The listing builds one solid part. Answer for the finished solid, in the listing's coordinates (mm). Round coordinates to 2 decimals unless told otherwise and drop trailing zeros. Write each loop counter-clockwise with the first axis right and the second up, starting at its lowest first coordinate (ties: lowest second). Pieces come first, ordered by that corner, then holes. Notation, with made-up numbers: M 10,89 L 21,89 A20 cw 21,126 Z; hole C 89,31 d5. An arc over 180 degrees is marked long. Write each question's results on one line, items separated by ' | '.
from build123d import *

# Parameters (mm, degrees)
F0_W     = 152.4
F0_H     = 152.4
F0_R     = 12.7
F1_DEPTH = 152.4
F2_R     = 15.0984188398
F2_R_2   = 23.2988824092
F2_R_3   = 22.4609439984
F2_R_4   = 13.2743249865
F3_DEPTH = 152.401


# Not quite as in the source:
# - the program builds the solid bodies; features that only make, move or delete a surface that nothing else refers to are left out


with BuildPart() as f1:
    # F0 (on Top) → F1 (new body)
    with BuildSketch(Plane.XY):
        Rectangle(F0_W, F0_H)
        Circle(F0_R, mode=Mode.SUBTRACT)
    extrude(amount=F1_DEPTH)

    # F2 (on face) → F3 (cut, through all)
    with BuildSketch(Plane.XZ.offset(76.2)):
        with Locations((-40.0141887367, 122.3329827189)):
            Circle(F2_R)
        with Locations((36.8730016053, 114.2153069377)):
            Circle(F2_R_2)
        with Locations((50.8471243083, 33.929079771)):
            Circle(F2_R_3)
        with Locations((-34.4802364707, 44.915728271)):
            Circle(F2_R_4)
    extrude(amount=-F3_DEPTH, mode=Mode.SUBTRACT)


solid = f1.part
1) Section D-D (x = 53.5) is taken. Determine the outline of the cut face in (y, z).
Return value:
outline: M -76.2,0 L 76.2,0 L 76.2,11.63 L -76.2,11.63 Z; M -76.2,56.23 L 76.2,56.23 L 76.2,97.89 L -76.2,97.89 Z; M -76.2,130.54 L 76.2,130.54 L 76.2,152.4 L -76.2,152.4 Z
2) Find the intervals of material crossed by line 1 (Z direction, x = 58, y = -60); line 2 (Z direction, x = 44.5, y = -11); line 3 (X direction, y = 17, z = 21), in increasing order.
Return value:
line 1: 0 to 12.64, 55.22 to 104.39, 124.04 to 152.4 | line 2: 0 to 12.38, 55.47 to 92.2, 136.23 to 152.4 | line 3: -76.2 to 32.48, 69.21 to 76.2
3) The mould has two halves that part along X. Classify faces 1 (the face through (-1, 76.2, 75)), 2 (the face through (-76.2, -1, 75)), 3 (the face through (-22.22, -1.07, 39.83)): +X half, -X half, draft (parallel to the pull), parting line (faces both ways), or undercut.
Return value:
face 1: draft | face 2: -X half | face 3: undercut
4) This flat-tipped pin is pushed along its axis until it touches: pin 1 (21 mm diameter, centred on x = -34.48, z = 44.92, fed in from -Y). Where does it stop, or does it pass through?
Return value:
pin 1: through
5) Section C-C (y = 0) is taken. Determine the outline of the cut face in (x, z).
Return value:
outline: M -76.2,0 L -12.7,0 L -12.7,152.4 L -76.2,152.4 Z; M 12.7,0 L 76.2,0 L 76.2,152.4 L 12.7,152.4 Z; hole C -40.01,122.33 d30.2; hole C -34.48,44.92 d26.55; hole C 36.87,114.22 d46.6; hole C 50.85,33.93 d44.92
6) Section A-A (z = 111) is taken. Determine the outline of the cut face in (x, y).
Return value:
outline: M -76.2,-76.2 L -49.99,-76.2 L -49.99,76.2 L -76.2,76.2 Z; M -30.04,-76.2 L 13.8,-76.2 L 13.8,76.2 L -30.04,76.2 Z; M 59.95,-76.2 L 76.2,-76.2 L 76.2,76.2 L 59.95,76.2 Z; hole C 0,0 d25.4
7) Section B-B (x = 0) is taken. Determine the outline of the cut face in (y, z).
Return value:
outline: M -76.2,0 L -12.7,0 L -12.7,152.4 L -76.2,152.4 Z; M 12.7,0 L 76.2,0 L 76.2,152.4 L 12.7,152.4 Z
